Geometry check sheet. Reference: the model listing, model coordinates, mm. Face numbers are marked on the shaded views. Give positions to 0.01 mm unless a question says otherwise; leave off trailing zeros. Write each loop counter-clockwise with the first axis right and the second up, starting at its lowest first coordinate (ties: lowest second). Pieces come first, ordered by that corner, then holes. Notation, with made-up numbers: (20, 16) - (72, 16) arc R7 ccw to (72, 28) - close; hole circle Ø1 at (83, -6.5). An arc over 180 degrees is marked (long way). One line per question, with ' | ' between items. Start each with the question number.
Q1. Section check C-C on x = 0. Record the boundary of the cut face in (y, z).
Q2. Section check D-D on x = -3.5. Record the boundary of the cut face in (y, z).
Q3. Section check B-B on y = 1.85. Record the boundary of the cut face in (x, z).
Q4. Release check for a two-part mould opening along X. For the marked faces 1, 2 and 3 record: +X half, -X half, draft (parallel to the pull), parting line (faces both ways), or undercut.
Q5. Thickness scan on L1, parallel to Z at x = 0, y = 1.65; L2, parallel to Y at x = 7, z = -13.75; L3, parallel to Z at x = -0.5, y = 1.3. Record the ranges inside material, lowest first. Write a range as [from, to].
Q6. Section check A-A on z = -18. Record the boundary of the cut face in (x, y), and give its area (3 significant figures).
Autodesk Inventor part; units mm, degrees
ref_plane "YZ Plane" through (0, 0, 0) normal (1, 0, 0) x (0, 1, 0)
ref_plane "XZ Plane" through (0, 0, 0) normal (0, 1, 0) x (-1, 0, 0)
ref_plane "XY Plane" through (0, 0, 0) normal (0, 0, 1) x (1, 0, 0)
sketch "スケッチ1" plane through (0, 0, 0) normal (0, 1, 0) x (-1, 0, 0)
  circle A0 centre (0, 0) radius 12.5
  line L0 (13, 0) -> (-13, 0)
  line L1 (-13, 0) -> (-13, -33)
  line L2 (-13, -33) -> (13, -33)
  line L3 (13, -33) -> (13, 0)
  circle A1 centre (0, 0) radius 16
  circle A2 centre (11, -31) radius 0.8
  circle A3 centre (-11, -31) radius 0.8
  circle A4 centre (0, -18) radius 0.8
  line L4 (0, -42.8) -> (0, 25.8)
  point P0 (13, -9.3274)
  point P1 (-13, -9.3274)
  point P2 (12.5, 0)
  point P3 (-12.5, 0)
  dimension "d0" = 25
  dimension "d1" = 26
  dimension "d2" = 33
  dimension "d3" = 32
  dimension "d9" = 1.6
  dimension "d10" = 1.6
  dimension "d11" = 2
  dimension "d12" = 2
  dimension "d13" = 2
  dimension "d14" = 2
  dimension "d15" = 1.6
  dimension "d16" = 15
extrude "押し出し1" add sketch "スケッチ1" along normal blind 3.75 contours L4 A4 L2 L1 A1 | A1 L3 L2 L4 A4
extrude "押し出し2" add sketch "スケッチ1" along normal blind 1.5 contours L0 L3 A1 L4 A0 | L4 A1 L1 L0 A0 picked at (2.1799, -14.5796) picked at (-2.1799, -14.5796)
fillet "フィレット1" radius 2 6 edges at (-13, 0.75, 0) (-12.5, 0.75, 0) (13, 0.75, 0) (12.5, 0.75, 0) (13, 1.875, -33) (-13, 1.875, -33)
properties part number "waist_cover"
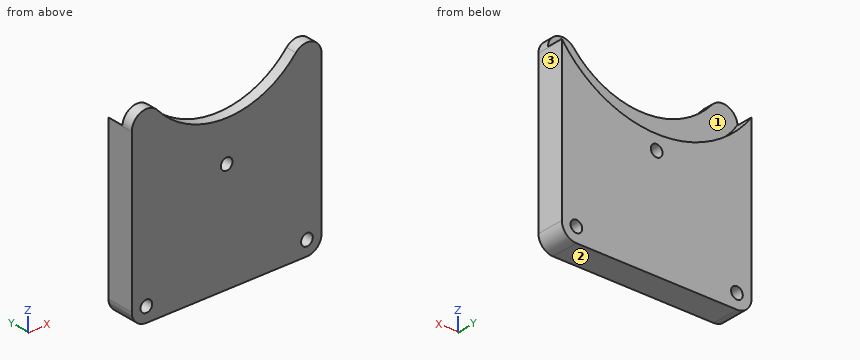
Working result:
1) outline: (0, -33) - (3.75, -33) - (3.75, -18.8) - (0, -18.8) - close; (0, -17.2) - (3.75, -17.2) - (3.75, -16) - (1.5, -16) - (1.5, -12.5) - (0, -12.5) - close
2) outline: (0, -33) - (3.75, -33) - (3.75, -15.61) - (1.5, -15.61) - (1.5, -12) - (0, -12) - close
3) outline: (-13, -31) arc R2 ccw to (-11, -33) - (11, -33) arc R2 ccw to (13, -31) - (13, -9.45) arc R2 ccw to (13, -9.33) arc R16 cw to (-13, -9.33) arc R2 ccw to (-13, -9.45) - close; hole circle Ø1.6 at (-11, -31); hole circle Ø1.6 at (0, -18); hole circle Ø1.6 at (11, -31)
4) face 1: undercut | face 2: draft | face 3: +X half
5) L1: z = [-33, -18.8], [-17.2, -16] | L2: y = [0, 1.5] | L3: z = [-33, -18.62], [-17.38, -12.49]
6) outline: (-13, 0) - (-0.8, 0) - (-0.8, 3.75) - (-13, 3.75) - close; (0.8, 0) - (13, 0) - (13, 3.75) - (0.8, 3.75) - close | area: 91.5 mm2
